Build history of the part. All positions in model axes, mm. Face numbers are marked on the shaded views. A direction names the side the tool comes from. Round coordinates to 2 decimals unless told otherwise and drop trailing zeros. Write each loop counter-clockwise with the first axis right and the second up, starting at its lowest first coordinate (ties: lowest second). Pieces come first, ordered by that corner, then holes. Notation, with made-up numbers: (-13, -5) - (42, -5) arc R18 cw to (42, 3) - close; hole circle Ø1 at (14.5, 23). An arc over 180 degrees is marked (long way). One line per question, with ' | ' between items.
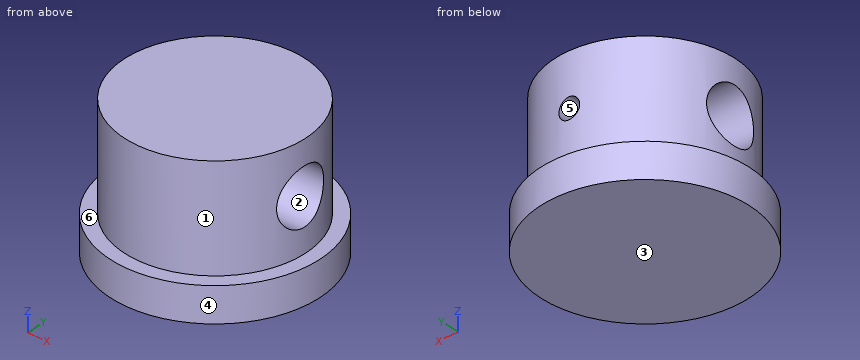
Autodesk Inventor part; units mm, degrees
ref_plane "YZ Plane" through (0, 0, 0) normal (1, 0, 0) x (0, 1, 0)
ref_plane "XZ Plane" through (0, 0, 0) normal (0, 1, 0) x (-1, 0, 0)
ref_plane "XY Plane" through (0, 0, 0) normal (0, 0, 1) x (1, 0, 0)
sketch "Szkic1" plane through (0, 0, 0) normal (0, 0, 1) x (1, 0, 0)
  circle A0 centre (0, 0) radius 15
  dimension "d0" = 30
extrude "Wyciągnięcie proste1" add sketch "Szkic1" along normal blind 5
sketch "Szkic2" plane through (0, 0, 5) normal (0, 0, 1) x (1, 0, 0)
  circle A0 centre (0, 0) radius 12.975
  dimension "d3" = 25.95
extrude "Wyciągnięcie proste2" add sketch "Szkic2" along normal blind 15
sketch "Szkic3" plane through (0, 0, 0) normal (0, 1, 0) x (-1, 0, 0)
  circle A0 centre (0, 12.5) radius 1.5
  point P0 (0, 0)
  dimension "d6" = 3
extrude "Wyciągnięcie proste3" cut sketch "Szkic3" along normal blind 20
thread "Gwint1"
sketch "Szkic4" plane through (0, 0, 0) normal (1, 0, 0) x (0, 1, 0)
  line L0 (0, 14) -> (0, 11)
  circle A0 centre (0, 12.5) radius 4
  point P0 (0, 0)
  dimension "d11" = 8
extrude "Wyciągnięcie proste4" cut sketch "Szkic4" along normal mid plane 35
properties part number "koncowka-wala" material "Aluminium 6061"
Q1. Saw through at A-A, the plane y = 0. List the corners of the cut face in (x, z) (3 decimals).
Found:
outline: (-15, 0) - (15, 0) - (15, 5) - (12.975, 5) - (12.975, 8.5) - (-12.975, 8.5) - (-12.975, 5) - (-15, 5) - close; (-12.975, 16.5) - (12.975, 16.5) - (12.975, 20) - (-12.975, 20) - close
Q2. Saw through at B-B, the plane x = 0. List the corners of the cut face in (y, z) (3 decimals), then the cut area to 3 significant figures.
Found:
outline: (-15, 0) - (15, 0) - (15, 5) - (12.975, 5) - (12.975, 11) - (3.708, 11) arc R4 cw (long way) to (3.708, 14) - (12.975, 14) - (12.975, 20) - (-12.975, 20) - (-12.975, 5) - (-15, 5) - close | area: 462 mm^2
Q3. Which spindle directions (+Z, -Z, +X, -X, +Y, -Y) get a long thin tool onto all of the face, cutting with end or side? Do the marked faces 4, 5 and 6. Say none if no direction does.
Found:
face 4: +Z, -Z | face 5: +Y | face 6: +Z
Q4. Drill centre lines: L1, parallel to Y at x = 0, z = 2; L2, parallel to Z at x = -13.25, y = 3.5; L3, parallel to Y at x = 2.75, z = 12.5. Where is each one in solid material? Low to high. Write a range as from..to.
Found:
L1: -15..15 | L2: 0..5 | L3: -12.68..-4, 4..12.68
Q5. Drop flat-ended pins along their axis: pin 1 (10 mm diameter, centred on x = 6.5, z = 3, fed in from +Y); pin 2 (1.5 mm diameter, centred on x = -10.5, z = 2, fed in from -Y); pin 3 (4 mm diameter, centred on x = 10.5, z = 11, fed in from -Y). Give the stop position or say it passes through.
Found:
pin 1: y = 14.92 | pin 2: y = -11.4 | pin 3: y = -9.8
Q6. Saw through at D-D, the plane x = 3.25. List the corners of the cut face in (y, z).
Found:
outline: (-14.64, 0) - (14.64, 0) - (14.64, 5) - (12.56, 5) - (12.56, 20) - (-12.56, 20) - (-12.56, 5) - (-14.64, 5) - close; hole circle Ø8 at (0, 12.5)
Q7. Pull direction Y, two halves, no side cores. Call the marked faces 1, 2 and 3: +Y half, -Y half, draft (parallel to the pull), parting line (faces both ways), or undercut.
Found:
face 1: parting line | face 2: undercut | face 3: draft
Q8. Saw through at C-C, the plane z = 12.5. List the corners of the cut face in (x, y) (3 decimals), then the cut area to 3 significant figures.
Found:
outline: (-12.343, -4) arc R12.975 ccw to (12.343, -4) - close; (-12.343, 4) - (-1.5, 4) - (-1.5, 12.888) arc R12.975 ccw to start; (1.5, 4) - (12.343, 4) arc R12.975 ccw to (1.5, 12.888) - close | area: 298 mm^2
